Could you check a few things on this model? Use its own coordinates, in mm. A direction names the side the tool comes from. Give positions to 0.01 mm unless a question says otherwise; leave off trailing zeros.
(1) Will these pins go through, and if not, where does the flat tip stop? pin 1 (5 mm diameter, centred on y = 15.875, z = 342.9, fed in from -X); pin 2 (1 mm diameter, centred on x = 26, z = 182, fed in from +Y) (3 decimals).
(2) If we mould it in two halves opening along X, with no side actions, what happens to faces 1 (the flat face through (3.175, 17, 263)), 2 (the flat face through (0, 16, 263)), 3 (the flat face through (31.75, 16, 263))? For each: released by +X, released by -X, zero draft, split by the parting line, or undercut.
(3) If I drill on probe 1 along X at (y, z) = (9, 33) (3 decimals); probe 2 along Y at (x, z) = (1.7, 215.9) (3 decimals); probe 3 along Y at (x, z) = (6.5, 438.5) (3 decimals), over which ranges is the centre line in solid material (lowest first)?
(4) On a 3-axis mill with a long thin cutter (end or side, diameter ignored), from which of +Z, -Z, +X, -X, +Y, -Y can I reach the whole of each face in a straight line? I mean faces 4 (the flat face through (16, 3, 533.4)), 5 (the flat face through (16, 3.175, 263)). Say none if no direction works.
Autodesk Inventor part; units mm, degrees
ref_plane "YZ Plane" through (0, 0, 0) normal (1, 0, 0) x (0, 1, 0)
ref_plane "XZ Plane" through (0, 0, 0) normal (0, 1, 0) x (-1, 0, 0)
ref_plane "XY Plane" through (0, 0, 0) normal (0, 0, 1) x (1, 0, 0)
sketch "Sketch1" plane through (0, 0, 0) normal (0, 0, 1) x (1, 0, 0)
  line L0 (3.175, 0) -> (28.575, 0)
  line L1 (31.75, 3.175) -> (31.75, 28.575)
  line L2 (0, 28.575) -> (0, 3.175)
  line L3 (4.7625, 3.175) -> (26.9875, 3.175)
  line L4 (28.575, 4.7625) -> (28.575, 28.575)
  line L5 (3.175, 28.575) -> (3.175, 4.7625)
  line L6 (0, 28.575) -> (3.175, 28.575)
  line L7 (28.575, 28.575) -> (31.75, 28.575)
  arc A0 (3.175, 4.7625) -> (4.7625, 3.175) centre (4.7625, 4.7625) ccw
  arc A1 (26.9875, 3.175) -> (28.575, 4.7625) centre (26.9875, 4.7625) ccw
  arc A2 (0, 3.175) -> (3.175, 0) centre (3.175, 3.175) ccw
  arc A3 (28.575, 0) -> (31.75, 3.175) centre (28.575, 3.175) ccw
  point P0 (0, 0)
  point P1 (0, 0)
  point P2 (31.75, 0)
  dimension "d0" = 31.75
  dimension "d1" = 28.575
  dimension "d2" = 1.5875
  dimension "d3" = 3.175
extrude "Extrusion1" add sketch "Sketch1" along normal blind 533.4
sketch "Sketch2" plane through (31.75, 3.175, 0) normal (1, 0, 0) x (0, 0, -1)
  line L0 (-533.4, 0) -> (-533.4, 25.4)
  line L1 (0, 0) -> (-533.4, 0)
  line L2 (-533.4, 12.7) -> (-520.7, 12.7)
  point P0 (0, -3.175)
  dimension "d6" = 12.7
hole "Hole1" at (31.75, 15.875, 520.7) direction (-1, 0, 0) diameter 6.35 end through all
sketch "Sketch3" plane through (3.175, 0, 0) normal (0, -1, 0) x (1, 0, 0)
  line L0 (0, 533.4) -> (25.4, 533.4)
  line L1 (0, 0) -> (0, 533.4)
  line L2 (12.7, 533.4) -> (12.7, 520.7)
  point P0 (-3.175, 0)
  dimension "d14" = 12.7
hole "Hole2" at (15.875, 0, 520.7) direction (0, 1, 0) diameter 6.35 end through all
pattern_linear "Rectangular Pattern1" count 21 spacing 25.4 along (0, 0, -1) of "Hole1", "Hole2"
properties part number "21 in bar"
Answer block:
1. pin 1: passes through
1. pin 2: stops at y = 3.175
2. face 1: undercut
2. face 2: released by -X
2. face 3: released by +X
3. probe 1: x = 0 to 3.175, 28.575 to 31.75
3. probe 2: y = 0.363 to 12.7, 19.05 to 28.575
3. probe 3: y = 0 to 3.175
4. face 4: +Z, +X, -X, +Y, -Y
4. face 5: +Z, -Z, +Y
